```python
from build123d import *

# Parameters (mm, degrees)
BOSS_EXTRUDE1_DEPTH     = 3.175
SKETCH2_R               = 1.905
CUT_EXTRUDE1_DEPTH      = 20.05
CUT_EXTRUDE1_DEPTH_BACK = 20.05


with BuildPart() as part:
    # Sketch1 → Boss-Extrude1 (new body, symmetric)
    with BuildSketch(Plane(origin=(0, 0, 0), x_dir=(1, 0, 0), z_dir=(0, 1, 0))):
        Polygon((-19.05, 28.623002286), (-19.05, 7.559996871), (-10.16, -28.655798535), (-6.35, -28.655798535), (-6.35, -15.955798535), (6.35, -15.955798535), (6.35, -28.655798535), (10.16, -28.655798535), (19.05, 7.559996871), (19.05, 28.623002286), (12.7, 28.623002286), (12.7, 15.923002286), (-12.7, 15.923002286), (-12.7, 28.623002286), align=None)
    extrude(amount=BOSS_EXTRUDE1_DEPTH, both=True)

    # Sketch2 → Cut-Extrude1 (cut, two sides)
    with BuildSketch(Plane.ZY) as cut_extrude1_sk:
        with Locations((-25.12220376, 0)):
            Circle(SKETCH2_R)
        with Locations((23.04976617, 0)):
            Circle(SKETCH2_R)
    extrude(amount=CUT_EXTRUDE1_DEPTH, mode=Mode.SUBTRACT)
    extrude(cut_extrude1_sk.sketch, amount=-CUT_EXTRUDE1_DEPTH_BACK, mode=Mode.SUBTRACT)


solid = part.part
```
Can you work these out from the model? Positions are in its coordinate system, mm. A direction names the side the tool comes from. Round coordinates to 2 decimals unless told otherwise and drop trailing zeros. Loops run counter-clockwise (first coordinate to the right, second up) from the corner with the lowest first, then second, coordinate; pieces in that order, holes last. Notation, with made-up numbers: M 31,-23 L 73,-23 A15 ccw 73,-3 Z; hole C 61,-36.5 d3. An arc over 180 degrees is marked long. Write item = value, one per line. Start each with the question number.
(1) Which directions (+Z, -Z, +X, -X, +Y, -Y) give clear straight access to the entire face, cutting with the end or side of a thin tool? Please do faces 1 (the face through (-6.35, 0.04, 20.98)), 2 (the face through (-16, 0, -28.623)), 3 (the face through (12.7, 0, -22)).
(2) Suppose I cut it at B-B on z = 19. Write out the boundary of the cut face in (x, y) (3 decimals).
(3) I need wall thicknesses on line 1 along X through (y, z) = (-2.25, -20); line 2 along X through (y, z) = (-1.25, 17.5); line 3 along Z through (x, y) = (-7.5, 0). Which ranges of each line are inside material? Lowest first, please.
(4) Suppose I cut it at A-A on y = 0. Give the number of separate pieces and of enclosed holes in the cut face, plus the area to 3 significant figures.
(5) Suppose I cut it at D-D on x = -16. Write out the boundary of the cut face in (y, z) (3 decimals).
(6) If we mould it in two halves opening along Z, with no side actions, what happens to faces 4 (the face through (-15.831, 0.084, -27.025)), 5 (the face through (16, 0, -28.623)), 6 (the face through (6.35, 0, 20.8)), 7 (the face through (8, 0, 28.656))? For each: released by +Z, released by -Z, zero draft, split by the parting line, or undercut.
(7) I'm going to push flat-ended pins straight in: P1, Ø3, axis at y = 0.5, z = 21.5, coming from the +X side; P2, Ø3, axis at x = 2.5, y = 1.5, coming from the +Z side; P3, Ø1.9, axis at x = 1, y = -1, coming from the -Z side. Where does each tip first touch, or does it pass through?
(8) Suppose I cut it at C-C on x = -8. Write out the boundary of the cut face in (y, z) (3 decimals), plus the area to 3 significant figures.
Answer block:
q1.face_1 = +Z, +Y, -Y
q1.face_2 = -Z, +X, -X, +Y, -Y
q1.face_3 = -Z, +Y, -Y
q2.outline = M -12.53,-3.175 L -6.35,-3.175 L -6.35,3.175 L -12.53,3.175 Z; M 6.35,-3.175 L 12.53,-3.175 L 12.53,3.175 L 6.35,3.175 Z
q3.line_1 = -19.05 to -12.7, 12.7 to 19.05
q3.line_2 = -12.9 to -6.35, 6.35 to 12.9
q3.line_3 = -15.92 to 21.14, 24.95 to 28.66
q4.separate_pieces = 5
q4.enclosed_holes = 0
q4.area = 1,290 mm²
q5.outline = M -3.175,-28.623 L 3.175,-28.623 L 3.175,4.865 L -3.175,4.865 Z; hole C 0,-25.122 d3.81
q6.face_4 = undercut
q6.face_5 = released by -Z
q6.face_6 = zero draft
q6.face_7 = released by +Z
q7.P1 = 12.28
q7.P2 = 15.96
q7.P3 = -15.92
q8.outline = M -3.175,-15.923 L 3.175,-15.923 L 3.175,28.656 L -3.175,28.656 Z; hole C 0,23.05 d3.81
q8.area = 272 mm²
